Verification items for the finished model (mm, model axes). Face numbers are marked on the shaded views. A direction names the side the tool comes from. Round coordinates to 2 decimals unless told otherwise and drop trailing zeros. Write each loop counter-clockwise with the first axis right and the second up, starting at its lowest first coordinate (ties: lowest second). Pieces come first, ordered by that corner, then holes. Notation, with made-up numbers: (89, -13) -> (101, -13) arc R32 ccw to (101, 15) -> close; hole circle Ø9 at (-28.75, -10.5). An arc over 180 degrees is marked (long way). Answer as a JSON object with one key per item and string values. Group by question number.
(1) Sectioned sample at A-A on y = 0. Record the cut outline in (x, z), and give its area (3 significant figures).
(2) Sectioned sample at C-C on z = 26.5. Record the cut outline in (x, y), and give its area (3 significant figures).
(3) Sectioned sample at D-D on z = 8. Record the cut outline in (x, y), and give its area (3 significant figures).
(4) Scan lines: L1, parallel to Z at x = 6.5, y = -2; L2, parallel to Y at x = 4.25, z = 16; L3, parallel to X at y = 1, z = 27.5. Record each from-to range of solid material in increasing order. Write a range as from..to.
(5) Set-up check for the marked faces 1 and 2: record each of +Z, -Z, +X, -X, +Y, -Y from which the full face is reachable in a straight line by a thin tool's end or side.
(6) Sectioned sample at B-B on x = 0. Record the cut outline in (y, z).
(7) Gauge pin test, flat ends, axial feed: pin 1 Ø10 at (y, z) = (-4.5, 23) entering from +X; pin 2 Ø6 at (x, z) = (-2.5, 25) entering from +Y; pin 3 Ø3 at (x, y) = (-3, 8.5) entering from +Z. Record the tip position at first contact, or that the pin passes through.
```python
from build123d import *

# Parameters (mm, degrees)
BOSS_EXTRUDE1_DEPTH = 10
SKETCH2_R           = 5
BOSS_EXTRUDE2_DEPTH = 25


with BuildPart() as part:
    # Sketch1 → Boss-Extrude1 (new body)
    with BuildSketch(Plane.XY):
        with BuildLine():
            Line((-0.580259609, 10.915085842), (3.385519837, 10.392981073))
            Line((3.385519837, 10.392981073), (2.99394126, 7.418646489))
            ThreePointArc((2.99394126, 7.418646489), (-1.044209538, -7.931558891), (-0.971838185, 7.940751258))
            Line((-0.971838185, 7.940751258), (-0.580259609, 10.915085842))
        make_face()
    extrude(amount=BOSS_EXTRUDE1_DEPTH)

    # Sketch2 → Boss-Extrude2 (add)
    with BuildSketch(Plane.XY.offset(10)):
        Circle(SKETCH2_R)
    extrude(amount=BOSS_EXTRUDE2_DEPTH)


solid = part.part
```
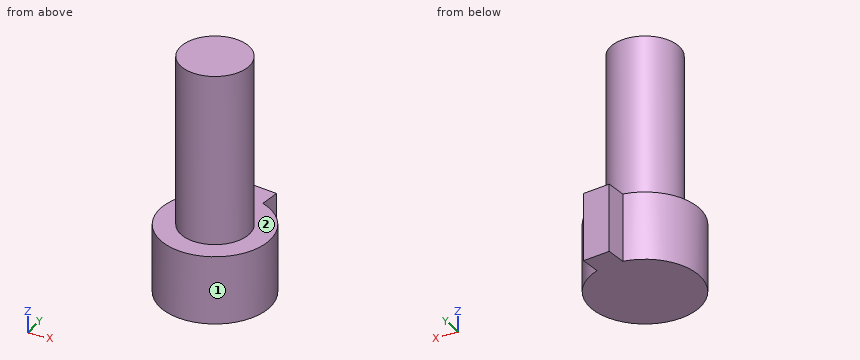
Computed values:
{
 "1": {"outline": "(-8, 0) -> (8, 0) -> (8, 10) -> (5, 10) -> (5, 35) -> (-5, 35) -> (-5, 10) -> (-8, 10) -> close", "area": "410 mm2"},
 "2": {"outline": "circle Ø10 at (0, 0)", "area": "78.5 mm2"},
 "3": {"outline": "(-0.97, 7.94) arc R8 ccw (long way) to (2.99, 7.42) -> (3.39, 10.39) -> (-0.58, 10.92) -> close", "area": "212 mm2"},
 "4": {"L1": "0..10", "L2": "-2.63..2.63", "L3": "-4.9..4.9"},
 "5": {"face 1": "+Z, -Z", "face 2": "+Z"},
 "6": {"outline": "(-8, 0) -> (10.84, 0) -> (10.84, 10) -> (5, 10) -> (5, 35) -> (-5, 35) -> (-5, 10) -> (-8, 10) -> close"},
 "7": {"pin 1": "x = 5", "pin 2": "y = 5", "pin 3": "z = 10"}
}
